Verification items for this drawing (mm, ordinates from the low corner). A direction names the side the tool comes from. Round coordinates to 2 decimals unless told otherwise and drop trailing zeros. Order: outer loops, then holes, each group sorted by start corner. A loop starts at its lowest first (then second) coordinate and runs counter-clockwise, first axis right, second up. Notation, with made-up numbers: (-16, 24) - (19, 24) arc R14 ccw to (19, 51) - close; hole circle Ø9 at (35.5, 36.5). An arc over 180 degrees is marked (long way). Use a Markdown table: item, result. Add a question column.
(1) Gauge pin test, flat ends, axial feed: P1, Ø0.6, axis at x = 25, y = 12.5, coming from the -Z side; P2, Ø3, axis at x = 9.5, z = 6.5, coming from the -Y side. Record the tip position at first contact, or that the pin passes through.
(2) Section check A-A on y = 4.25. Record the boundary of the cut face in (x, z), then the cut area to 3 significant figures.
(3) Section check B-B on x = 2.5. Record the boundary of the cut face in (y, z).
(4) Section check D-D on z = 5. Record the boundary of the cut face in (x, y).
(5) Thickness scan on line 1 along X through (y, z) = (7, 4); line 2 along X through (y, z) = (10.75, 4); line 3 along Z through (x, y) = (30, 5.5). Record the ranges inside material, lowest first. Write a range as [from, to].
(6) Access from +Z, -Z, +X, -X, +Y, -Y to the whole of each face (thin tool, end or side, straight path). Record for the marked faces 1, 2 and 3.
(7) Mould release check, pull along X, two halves, no side actions. Record for the marked faces 4, 5, 6 and 7: released by +X, released by -X, zero draft, split by the parting line, or undercut.
(8) Section check C-C on z = 1.75. Record the boundary of the cut face in (x, y), then the cut area to 3 significant figures.
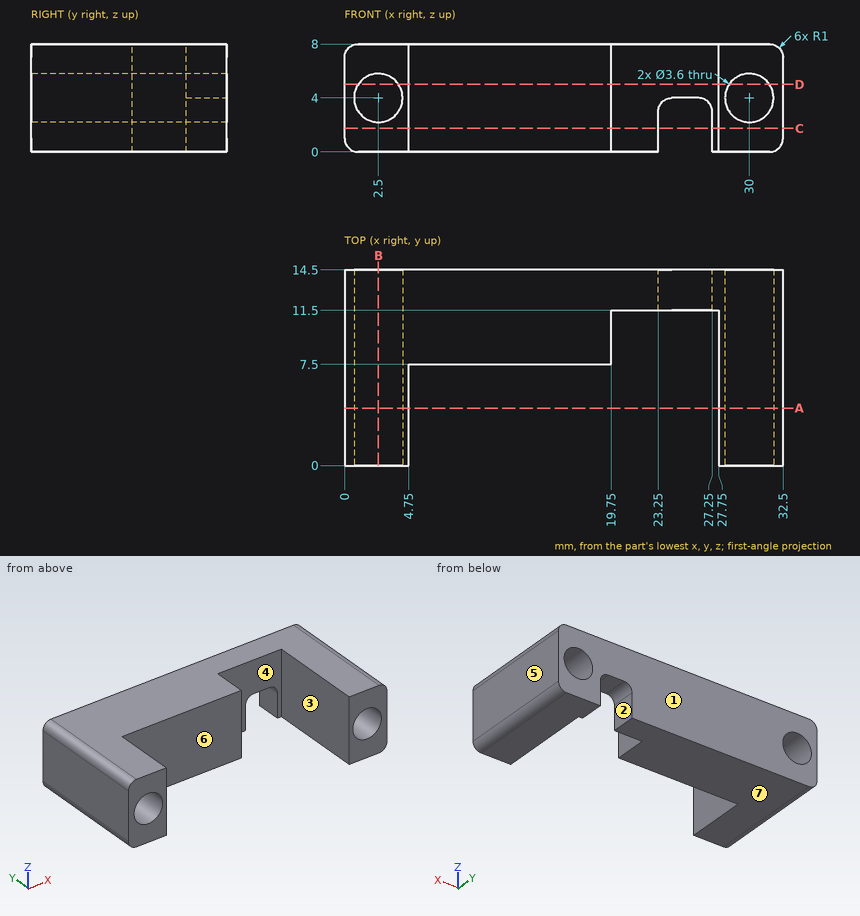
Check sheet entries:
| question | item | result |
|---|---|---|
| 1 | P1 | stops at z = 4 |
| 1 | P2 | stops at y = 7.5 |
| 2 | outline | (0, 1) arc R1 ccw to (1, 0) - (4.75, 0) - (4.75, 8) - (1, 8) arc R1 ccw to (0, 7) - close; (27.75, 0) - (31.5, 0) arc R1 ccw to (32.5, 1) - (32.5, 7) arc R1 ccw to (31.5, 8) - (27.75, 8) - close; hole circle Ø3.6 at (2.5, 4); hole circle Ø3.6 at (30, 4) |
| 2 | area | 54.8 mm2 |
| 3 | outline | (0, 0) - (14.5, 0) - (14.5, 2.2) - (0, 2.2) - close; (0, 5.8) - (14.5, 5.8) - (14.5, 8) - (0, 8) - close |
| 4 | outline | (0, 0) - (1, 0) - (1, 14.5) - (0, 14.5) - close; (4, 0) - (4.75, 0) - (4.75, 7.5) - (19.75, 7.5) - (19.75, 11.5) - (27.75, 11.5) - (27.75, 0) - (28.5, 0) - (28.5, 14.5) - (4, 14.5) - close; (31.5, 0) - (32.5, 0) - (32.5, 14.5) - (31.5, 14.5) - close |
| 5 | line 1 | x = [0, 0.7], [4.3, 4.75], [27.75, 28.2], [31.8, 32.5] |
| 5 | line 2 | x = [0, 0.7], [4.3, 19.75], [27.75, 28.2], [31.8, 32.5] |
| 5 | line 3 | z = [0, 2.2], [5.8, 8] |
| 6 | face 1 | +Z, -Z, +X, -X, +Y |
| 6 | face 2 | -Z, +Y, -Y |
| 6 | face 3 | +Z, -Z, -Y |
| 7 | face 4 | undercut |
| 7 | face 5 | released by +X |
| 7 | face 6 | undercut |
| 7 | face 7 | zero draft |
| 8 | outline | (0, 0) - (4.75, 0) - (4.75, 7.5) - (19.75, 7.5) - (19.75, 11.5) - (23.25, 11.5) - (23.25, 14.5) - (0, 14.5) - close; (27.25, 11.5) - (27.75, 11.5) - (27.75, 0) - (32.5, 0) - (32.5, 14.5) - (27.25, 14.5) - close |
| 8 | area | 255 mm2 |
